from build123d import *

# Parameters (mm, degrees)
SKETCH1_R           = 5
BOSS_EXTRUDE1_DEPTH = 80
CUT_EXTRUDE1_DEPTH  = 15
SKETCH3_R           = 2
CUT_EXTRUDE2_DEPTH  = 81.554329493


with BuildPart() as part:
    # Sketch1 → Boss-Extrude1 (new, symmetric)
    with BuildSketch(Plane(origin=(0, 0, 0), x_dir=(1, 0, 0), z_dir=(0, 1, 0))):
        with Locations(Location((0, 0, 0), (0, 0, 270))):
            Circle(SKETCH1_R)
    extrude(amount=BOSS_EXTRUDE1_DEPTH, both=True)

    # Sketch2 → Cut-Extrude1 (cut)
    with BuildSketch(Plane(origin=(0, 80, 0), x_dir=(1, 0, 0), z_dir=(0, 1, 0))):
        with BuildLine():
            Line((-4, -3), (4, -3))
            ThreePointArc((4, -3), (0, -5), (-4, -3))
        make_face()
        with BuildLine():
            Line((-4, 3), (4, 3))
            ThreePointArc((4, 3), (0, 5), (-4, 3))
        make_face()
    cut_extrude1 = extrude(amount=-CUT_EXTRUDE1_DEPTH, mode=Mode.SUBTRACT)

    # Mirror2: Cut-Extrude1 across plane
    add(cut_extrude1.mirror(Plane.ZX), mode=Mode.SUBTRACT)

    # Sketch3 → Cut-Extrude2 (cut, through all)
    with BuildSketch(Plane.XY.offset(3)):
        with Locations((0, 74)):
            Circle(SKETCH3_R)
    cut_extrude2 = extrude(amount=-CUT_EXTRUDE2_DEPTH, mode=Mode.SUBTRACT)

    # Mirror3: Cut-Extrude2 across plane
    add(cut_extrude2.mirror(Plane.ZX), mode=Mode.SUBTRACT)


solid = part.part
The listing builds one solid part. Answer for the finished solid, in the listing's coordinates (mm). A direction names the side the tool comes from. Coordinates: 2 decimals unless noted, no trailing zeros. Write each loop counter-clockwise with the first axis right and the second up, starting at its lowest first coordinate (ties: lowest second). Pieces come first, ordered by that corner, then holes. Notation, with made-up numbers: (-4.75, 0) -> (13.25, 0) arc R28 ccw to (13.25, 25) -> close; hole circle Ø10 at (-30.5, 48). An arc over 180 degrees is marked (long way). One line per question, with ' | ' between items.
1. Section C-C (z = 0) is taken. Determine the outline of the cut face in (x, y), and give its area (3 significant figures).
Verdict:
outline: (-5, -80) -> (5, -80) -> (5, 80) -> (-5, 80) -> close; hole circle Ø4 at (0, -74); hole circle Ø4 at (0, 74) | area: 1,570 mm^2
2. Section D-D (y = 23) is taken. Determine the outline of the cut face in (x, z), and give its area (3 significant figures).
Verdict:
outline: circle Ø10 at (0, 0) | area: 78.5 mm^2
3. Section B-B (y = 74) is taken. Determine the outline of the cut face in (x, z), and give its area (3 significant figures).
Verdict:
outline: (-4, -3) -> (-2, -3) -> (-2, 3) -> (-4, 3) arc R5 ccw to start; (2, -3) -> (4, -3) arc R5 ccw to (4, 3) -> (2, 3) -> close | area: 32.2 mm^2
4. Section A-A (x = 0) is taken. Determine the outline of the cut face in (y, z), and give its area (3 significant figures).
Verdict:
outline: (-80, -3) -> (-76, -3) -> (-76, 3) -> (-80, 3) -> close; (-72, -3) -> (-65, -3) -> (-65, -5) -> (65, -5) -> (65, -3) -> (72, -3) -> (72, 3) -> (65, 3) -> (65, 5) -> (-65, 5) -> (-65, 3) -> (-72, 3) -> close; (76, -3) -> (80, -3) -> (80, 3) -> (76, 3) -> close | area: 1,430 mm^2
5. Straight lines are drawn through the part: line 1 (Y direction, x = 0, z = -1.6); line 2 (Y direction, x = 0.75, z = -2.25); line 3 (Z direction, x = 3, y = -65.5). For each, find the intervals that lie inside material, in ascending order.
Verdict:
line 1: y = -80 to -76, -72 to 72, 76 to 80 | line 2: y = -80 to -75.85, -72.15 to 72.15, 75.85 to 80 | line 3: z = -3 to 3
6. Which of the six approach directions +Z, -Z, +X, -X, +Y, -Y give full straight-line access (tool end or side, diameter ignored) to faces 1 (the flat face through (0, 71, 3)), 2 (the cylindrical face through (0, 76, 0)), 3 (the flat face through (0, -71, -3)), 4 (the flat face through (0, 71, -3)), 5 (the flat face through (0, -71, 3))?
Verdict:
face 1: +Z, +X, -X, +Y | face 2: +Z, -Z | face 3: -Z, +X, -X, -Y | face 4: -Z, +X, -X, +Y | face 5: +Z, +X, -X, -Y
7. Given pin 1 Ø1 at (x, z) = (1.5, 4.5) entering from -Y; pin 2 Ø4 at (x, y) = (0, -69.5) entering from -Z; pin 3 Ø2 at (y, z) = (27, 1.5) entering from -X; pin 4 Ø3 at (x, y) = (0, 74) entering from +Z, each flat-ended and moving along its own axis, determine where each tip first touches the part or whether it passes through.
Verdict:
pin 1: stops at y = -65 | pin 2: stops at z = -3 | pin 3: stops at x = -4.97 | pin 4: passes through
8. For a pull along Y with two mould halves and no side action, classify faces 6 (the flat face through (0, -80, 0)), 7 (the cylindrical face through (0, -76, 0)), 8 (the flat face through (0, 80, 0)), 9 (the cylindrical face through (1.5, 1.12, 4.77)) as released by +Y, released by -Y, zero draft, split by the parting line, or undercut.
Verdict:
face 6: released by -Y | face 7: undercut | face 8: released by +Y | face 9: zero draft
